Design review of the part built by this model. Coordinates are the model's own, in mm. Face numbers are marked on the shaded views. A direction names the side the tool comes from. Coordinates: 2 decimals unless noted, no trailing zeros. Order: outer loops, then holes, each group sorted by start corner. A loop starts at its lowest first (then second) coordinate and runs counter-clockwise, first axis right, second up. Notation, with made-up numbers: (77.5, -14) -> (97.5, -14) arc R19 cw to (97.5, 15) -> close; hole circle Ø8 at (71.25, -19). An arc over 180 degrees is marked (long way). Write item = value, one per line.
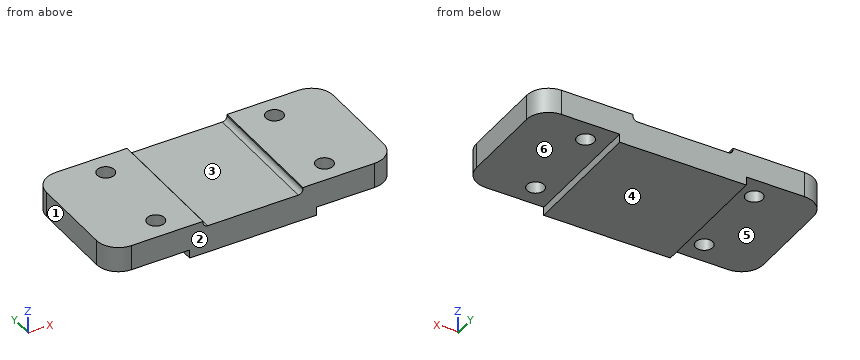
```python
from build123d import *

# Parameters (mm, degrees)
F1_DEPTH = 82
F2_R     = 14
F3_R     = 5.5
F4_DEPTH = 21.610834


with BuildPart() as f1:
    # F0 (on Front) → F1 (new body)
    with BuildSketch(Plane.XZ):
        with BuildLine():
            Line((0, 21.609834), (0, 5.402458))
            Line((0, 5.402458), (51.323355, 5.402458))
            Line((51.323355, 5.402458), (51.323355, 0))
            Line((51.323355, 0), (132.360232, 0))
            Line((132.360232, 0), (132.360232, 5.402458))
            Line((132.360232, 5.402458), (183.683587, 5.402458))
            Line((183.683587, 5.402458), (183.683587, 21.609834))
            Line((183.683587, 21.609834), (123.841794, 21.609834))
            Line((123.841794, 21.609834), (123.841794, 20.609834))
            ThreePointArc((123.841794, 20.609834), (122.963114, 18.488513), (120.841794, 17.609834))
            Line((120.841794, 17.609834), (62.875107, 17.609834))
            ThreePointArc((62.875107, 17.609834), (60.787768, 18.455068), (59.876622, 20.514491))
            Line((59.876622, 20.514491), (59.841794, 21.609834))
            Line((59.841794, 21.609834), (0, 21.609834))
        make_face()
    extrude(amount=F1_DEPTH)

    # F2
    f2_edges = [f1.edges().sort_by_distance(p)[0] for p in [
        (0, -82, 13.506146),
        (183.683587, -82, 13.506146),
        (183.683587, 0, 13.506146),
        (0, 0, 13.506146),
    ]]
    fillet(f2_edges, radius=F2_R)

    # F3 (on face) → F4 (cut, through all)
    with BuildSketch(Plane.XY.offset(21.609834)):
        with Locations((37.919445, -14)):
            Circle(F3_R)
        with Locations((145.919445, -14)):
            Circle(F3_R)
        with Locations((145.919445, -68)):
            Circle(F3_R)
        with Locations((37.919445, -68)):
            Circle(F3_R)
    extrude(amount=-F4_DEPTH, mode=Mode.SUBTRACT)


solid = f1.part
```
(1) We need section B-B (z = 11). Write out the cut boundary in (x, y).
Report:
outline = (0, -68) arc R14 ccw to (14, -82) -> (169.68, -82) arc R14 ccw to (183.68, -68) -> (183.68, -14) arc R14 ccw to (169.68, 0) -> (14, 0) arc R14 ccw to (0, -14) -> close; hole circle Ø11 at (37.92, -68); hole circle Ø11 at (37.92, -14); hole circle Ø11 at (145.92, -68); hole circle Ø11 at (145.92, -14)
(2) Insertion check: pin 1 (2 mm diameter, centred on y = -55, z = 4.5, fed in from -X); pin 2 (10 mm diameter, centred on x = 145.92, y = -14, fed in from +Z); pin 3 (17.5 mm diameter, centred on x = 37.92, y = -14, fed in from -Z); pin 4 (4.5 mm diameter, centred on y = -40, z = 2, fed in from -X). Each pin has a flat end and moves straight along its axis. Give the tip position at first contact, or say it passes through.
Report:
pin_1 = 0
pin_2 = through
pin_3 = 5.4
pin_4 = 51.32
(3) We need section C-C (y = -30.5). Write out the cut boundary in (x, z), and give its area (3 significant figures).
Report:
outline = (0, 5.4) -> (51.32, 5.4) -> (51.32, 0) -> (132.36, 0) -> (132.36, 5.4) -> (183.68, 5.4) -> (183.68, 21.61) -> (123.84, 21.61) -> (123.84, 20.61) arc R3 cw to (120.84, 17.61) -> (62.88, 17.61) arc R3 cw to (59.88, 20.51) -> (59.84, 21.61) -> (0, 21.61) -> close
area = 3,160 mm²
(4) For L1, parallel to X at y = -13.5, z = 7.5; L2, parallel to X at y = -18.5, z = 15.25; L3, parallel to Z at x = 23.5, y = -19.5, list the stretches that pass through material, from the lowest coordinate up.
Report:
L1 = 0.01 to 32.44, 43.4 to 140.44, 151.4 to 183.67
L2 = 0 to 34.76, 41.08 to 142.76, 149.08 to 183.68
L3 = 5.4 to 21.61
(5) We need section A-A (y = -17.5). Write out the cut boundary in (x, z), and give its area (3 significant figures).
Report:
outline = (0, 5.4) -> (33.68, 5.4) -> (33.68, 21.61) -> (0, 21.61) -> close; (42.16, 5.4) -> (51.32, 5.4) -> (51.32, 0) -> (132.36, 0) -> (132.36, 5.4) -> (141.68, 5.4) -> (141.68, 21.61) -> (123.84, 21.61) -> (123.84, 20.61) arc R3 cw to (120.84, 17.61) -> (62.88, 17.61) arc R3 cw to (59.88, 20.51) -> (59.84, 21.61) -> (42.16, 21.61) -> close; (150.16, 5.4) -> (183.68, 5.4) -> (183.68, 21.61) -> (150.16, 21.61) -> close
area = 2,890 mm²
(6) We need section D-D (x = 136). Write out the cut boundary in (y, z).
Report:
outline = (-82, 5.4) -> (0, 5.4) -> (0, 21.61) -> (-82, 21.61) -> close
(7) For the marked faces 4, 5 and 6, list the 3-axis set-ups (+Z, -Z, +X, -X, +Y, -Y) from which the entire face can be reached by the end or side of a thin tool; tool diameter is ignored.
Report:
face_4 = -Z, +X, -X, +Y, -Y
face_5 = -Z, -X, +Y, -Y
face_6 = -Z, +X, +Y, -Y
(8) The part is to be moulded in two halves that separate along X. For the marked faces 1, 2 and 3, say which applies: released by +X, released by -X, zero draft, split by the parting line, or undercut.
Report:
face_1 = released by -X
face_2 = zero draft
face_3 = undercut
